from build123d import *

# Parameters (mm, degrees)
BOSS_EXTRUDE1_DEPTH = 9
FILLET1_R           = 6
FILLET2_R           = 4
BOSS_EXTRUDE2_DEPTH = 18
LPATTERN1_COUNT     = 6
LPATTERN1_PITCH     = 6
CUT_EXTRUDE1_DEPTH  = 26
CUT_EXTRUDE2_DEPTH  = 8
SKETCH7_R           = 1.5
CUT_EXTRUDE3_DEPTH  = 26
SKETCH8_R           = 1.75
BOSS_EXTRUDE3_DEPTH = 3
SKETCH9_R           = 1.25
CUT_EXTRUDE4_DEPTH  = 1
SKETCH10_R          = 1.25
CUT_EXTRUDE5_DEPTH  = 1
CUT_EXTRUDE6_DEPTH  = 1


with BuildPart() as part:
    # Sketch2 → Boss-Extrude1 (new, symmetric)
    with BuildSketch(Plane(origin=(0, 0, 0), x_dir=(1, 0, 0), z_dir=(0, 1, 0))):
        with BuildLine():
            ThreePointArc((9.952664911, -63.474262908), (18.884876985, -63.429469216), (17.963436499, -72.314139521))
            Line((17.963436499, -72.314139521), (9.870678178, -78.188427797))
            Line((9.870678178, -78.188427797), (9.870678178, -128.188427797))
            Line((9.870678178, -128.188427797), (-1.129321822, -128.188427797))
            Line((-1.129321822, -128.188427797), (-1.129321822, -121.188427797))
            Line((-1.129321822, -121.188427797), (-9.195214577, -92.293075678))
            Line((-9.195214577, -92.293075678), (-19.97492157, -85.026858152))
            Line((-19.97492157, -85.026858152), (-16.951577323, -75.494838976))
            Line((-16.951577323, -75.494838976), (-11.784410902, -73.871887989))
            Line((-11.784410902, -73.871887989), (-2.640867258, -71))
            Line((-2.640867258, -71), (3.643526088, -70.578297923))
            Line((3.643526088, -70.578297923), (9.952664911, -63.474262908))
        make_face()
        Polygon((-11.784410902, -73.871887989), (-26.326484906, -3.871887989), (-2.640867258, 0), (-2.640867258, -71), align=None)
    extrude(amount=BOSS_EXTRUDE1_DEPTH, both=True)

    # Fillet1
    fillet1_edges = [part.edges().sort_by_distance(p)[0] for p in [
        (-26.326484906, 0, 3.871887989),
        (-2.640867258, 0, 0),
    ]]
    fillet(fillet1_edges, radius=FILLET1_R)

    # Fillet2
    fillet2_edges = [part.edges().sort_by_distance(p)[0] for p in [
        (-1.129321822, 0, 128.188427797),
        (-19.97492157, 0, 85.026858152),
        (-16.951577323, 0, 75.494838976),
    ]]
    fillet(fillet2_edges, radius=FILLET2_R)

    # Sketch3 → Boss-Extrude2 (add)
    with BuildSketch(Plane(origin=(0, 9, 0), x_dir=(1, 0, 0), z_dir=(0, 1, 0))):
        Polygon((9.870678178, -125.188427797), (9.870678178, -121.188427797), (13.870678178, -123.188427797), align=None)
    boss_extrude2 = extrude(amount=-BOSS_EXTRUDE2_DEPTH)

    # LPattern1: Boss-Extrude2 ×6
    with Locations(*[(0, 0, -i * LPATTERN1_PITCH) for i in range(1, LPATTERN1_COUNT)]):
        add(boss_extrude2)

    # Sketch5 → Cut-Extrude1 (cut)
    with BuildSketch(Plane(origin=(0, 9, 0), x_dir=(1, 0, 0), z_dir=(0, 1, 0))):
        Polygon((8.581909731, -96.366546328), (-6.418090269, -96.366546328), (8.581909731, -121.366546328), align=None)
    extrude(amount=-CUT_EXTRUDE1_DEPTH, mode=Mode.SUBTRACT)

    # Sketch6 → Cut-Extrude2 (cut)
    with BuildSketch(Plane(origin=(-32.431019942, 0, 9.052844475), x_dir=(0.2688630918299989, 0, 0.9631784039582769), z_dir=(-0.963178403958277, 0, 0.2688630918299989))):
        Polygon((93.422443507, 6), (93.422443507, -6), (111.422443507, -4.533928271), (111.422443507, 4.533928271), align=None)
    extrude(amount=-CUT_EXTRUDE2_DEPTH, mode=Mode.SUBTRACT)

    # Sketch7 → Cut-Extrude3 (cut)
    with BuildSketch(Plane(origin=(0, 9, 0), x_dir=(1, 0, 0), z_dir=(0, 1, 0))):
        with Locations(Location((-19.178129346, -8.782985081, 0), (0, 0, 270))):
            Circle(SKETCH7_R)
    extrude(amount=-CUT_EXTRUDE3_DEPTH, mode=Mode.SUBTRACT)

    # Sketch8 → Boss-Extrude3 (add)
    with BuildSketch(Plane(origin=(0, 9, 0), x_dir=(1, 0, 0), z_dir=(0, 1, 0))):
        with Locations(Location((14.438863534, -67.458484528, 0), (0, 0, 270))):
            Circle(SKETCH8_R)
        with Locations(Location((-15.257160901, -83.38305422, 0), (0, 0, 270))):
            Circle(SKETCH8_R)
    boss_extrude3 = extrude(amount=BOSS_EXTRUDE3_DEPTH)

    # Sketch9 → Cut-Extrude4 (cut)
    with BuildSketch(Plane(origin=(0, 12, 0), x_dir=(1, 0, 0), z_dir=(0, 1, 0))):
        with Locations(Location((-15.257160901, -83.38305422, 0), (0, 0, 270))):
            Circle(SKETCH9_R)
    cut_extrude4 = extrude(amount=-CUT_EXTRUDE4_DEPTH, mode=Mode.SUBTRACT)

    # Sketch10 → Cut-Extrude5 (cut)
    with BuildSketch(Plane(origin=(0, 12, 0), x_dir=(1, 0, 0), z_dir=(0, 1, 0))):
        with Locations(Location((14.438863534, -67.458484528, 0), (0, 0, 270))):
            Circle(SKETCH10_R)
    cut_extrude5 = extrude(amount=-CUT_EXTRUDE5_DEPTH, mode=Mode.SUBTRACT)

    # Sketch11 → Cut-Extrude6 (cut)
    with BuildSketch(Plane(origin=(0, 9, 0), x_dir=(1, 0, 0), z_dir=(0, 1, 0))):
        with BuildLine():
            Line((-15.375345178, -17.642535787), (-5.588816332, -66.731764476))
            ThreePointArc((-5.588816332, -66.731764476), (-7.046968284, -68.91608772), (-9.231291528, -67.457935767))
            Line((-9.231291528, -67.457935767), (-19.017820373, -18.368707078))
            ThreePointArc((-19.017820373, -18.368707078), (-17.559668421, -16.184383835), (-15.375345178, -17.642535787))
        make_face()
    cut_extrude6 = extrude(amount=-CUT_EXTRUDE6_DEPTH, mode=Mode.SUBTRACT)

    # Mirror1: Boss-Extrude3, Cut-Extrude4, Cut-Extrude5, Cut-Extrude6 across plane
    add(boss_extrude3.mirror(Plane.ZX))
    add(cut_extrude4.mirror(Plane.ZX), mode=Mode.SUBTRACT)
    add(cut_extrude5.mirror(Plane.ZX), mode=Mode.SUBTRACT)
    add(cut_extrude6.mirror(Plane.ZX), mode=Mode.SUBTRACT)


solid = part.part
The listing builds one solid part. Answer for the finished solid, in the listing's coordinates (mm). A direction names the side the tool comes from. Coordinates: 2 decimals unless noted, no trailing zeros. Loops run counter-clockwise (first coordinate to the right, second up) from the corner with the lowest first, then second, coordinate; pieces in that order, holes last. Notation, with made-up numbers: M -28,44 L -17,44 A31 ccw -17,80 Z; hole C 72.25,12 d5. An arc over 180 degrees is marked long. Answer in a Markdown table with one row per item.
1) Which of the six approach directions +Z, -Z, +X, -X, +Y, -Y give full straight-line access (tool end or side, diameter ignored) to faces 4 (the cylindrical face through (-15.736, 11.507, 84.538)), 5 (the flat face through (11.899, 0.126, 112.174)), 6 (the cylindrical face through (14.52, -10.48, 65.71))?
Answers below:
| item | result |
|---|---|
| face 4 | +Y |
| face 5 | +X, +Y, -Y |
| face 6 | -Y |
2) Determine the mould class of faces 1 (the cylindrical face through (14.52, 10.48, 65.71)), 2 (the flat face through (9.871, 0, 127)), 3 (the flat face through (-12, 8, 42)) for opening direction Z: released by +Z, released by -Z, zero draft, split by the parting line, or undercut.
Answers below:
| item | result |
|---|---|
| face 1 | split by the parting line |
| face 2 | zero draft |
| face 3 | undercut |
3) Find section B-B (z = 44.5). Determine the outline of the cut face in (x, y), then the cut area to 3 significant figures.
Answers below:
| item | result |
|---|---|
| outline | M -17.89,-9 L -13.81,-9 L -13.81,-8 L -10.02,-8 L -10.02,-9 L -2.64,-9 L -2.64,9 L -10.02,9 L -10.02,8 L -13.81,8 L -13.81,9 L -17.89,9 Z |
| area | 267 mm^2 |
4) Find the intervals of material crossed by probe 1 along Y at (x, z) = (-9, 22); probe 2 along X at (y, z) = (-2.25, 83); probe 3 along Z at (x, y) = (3, -1.5), in increasing order.
Answers below:
| item | result |
|---|---|
| probe 1 | -9 to 9 |
| probe 2 | -19.24 to 9.87 |
| probe 3 | 70.62 to 96.37, 114.84 to 128.19 |
5) Find section D-D (z = 80). Determine the outline of the cut face in (x, y).
Answers below:
| item | result |
|---|---|
| outline | M -18.38,-9 L 9.87,-9 L 9.87,9 L -18.38,9 Z |
6) Find section C-C (z = 58). Determine the outline of the cut face in (x, y).
Answers below:
| item | result |
|---|---|
| outline | M -15.08,-9 L -11.12,-9 L -11.12,-8 L -7.33,-8 L -7.33,-9 L -2.64,-9 L -2.64,9 L -7.33,9 L -7.33,8 L -11.12,8 L -11.12,9 L -15.08,9 Z |
7) Given pin 1 (4 mm diameter, centred on y = -2, z = 82.5, fed in from +X); pin 2 (8 mm diameter, centred on y = 5, z = 50, fed in from +X); pin 3 (0.7 mm diameter, centred on x = -15.5, z = 84, fed in from -Y); pin 4 (6 mm diameter, centred on x = 12.5, y = 9, fed in from +Z), each flat-ended and moving along its own axis, determine where each tip first touches the part or whether it passes through.
Answers below:
| item | result |
|---|---|
| pin 1 | x = 9.87 |
| pin 2 | x = -2.64 |
| pin 3 | y = -11 |
| pin 4 | z = 128.19 |
8) Find section A-A (x = 0.5). Determine the outline of the cut face in (y, z), then the cut area to 3 significant figures.
Answers below:
| item | result |
|---|---|
| outline | M -9,70.79 L 9,70.79 L 9,96.37 L -9,96.37 Z; M -9,107.9 L -5.13,107.9 L -4.53,115.54 L 4.53,115.54 L 5.13,107.9 L 9,107.9 L 9,127.41 L -9,127.41 Z |
| area | 738 mm^2 |
